Geometry: final body of the model. Coordinates: model frame, mm. A direction names the side the tool comes from. Give positions to 0.01 mm unless a question says otherwise; leave off trailing zeros. Write each loop counter-clockwise with the first axis right and the second up, starting at its lowest first coordinate (ties: lowest second). Pieces come first, ordered by that corner, then holes. Notation, with made-up numbers: (-40, -39) - (-17, -39) arc R28 cw to (-17, -5) - close; hole circle Ø3 at (80, 13.5). An arc over 180 degrees is marked (long way). Use CSV: the item, a comma, the result in double quotes. Start each with the question number.
(1) Line query: probe 1 along Y at (x, z) = (1, 2.3); probe 2 along Y at (x, z) = (3, 0.7); probe 3 along X at (y, z) = (-10.5, 3.85). Output: solid intervals per line, ascending. Write a range as [from, to].
(2) First-contact query: pin 1 Ø12 at (x, y) = (1.5, 9) entering from +Z. Flat tip, straight axial feed; report the tip coordinate or a pass-through.
(3) Draft query along Y for faces 3 (the flat face through (0, 0, 0)), 4 (the cylindrical face through (12.715, 12.699, 2.024)), 5 (the cylindrical face through (3.13, 10.81, 1.98)). Return one class per face: released by +Y, released by -Y, zero draft, split by the parting line, or undercut.
(4) Reachability of faces 1 (the flat face through (0, 13, 2)), 2 (the flat face through (0, 11.2, 2)) from +Z, -Z, +X, -X, +Y, -Y: full face, straight path, thin tool, end or side. Return the list, or none.
(5) Section B-B on x = 0. Output: boundary loops of the cut face in (y, z).
from build123d import *

# Parameters (mm, degrees)
F0_W     = 26
F0_H     = 26
F1_DEPTH = 4
F2_R     = 1
F4_W     = 7
F4_H     = 2.6
F5_DEPTH = 25
F6_R     = 1.29999
F7_R     = 0.3


# Not quite as in the source:
# - a fillet or chamfer is up to 0.001 mm smaller than in the source, because OpenCascade refuses the exact size


with BuildPart() as f1:
    # F0 (on Top) → F1 (new body)
    with BuildSketch(Plane.XY):
        Rectangle(F0_W, F0_H)
    extrude(amount=F1_DEPTH)

    # F2
    f2_edges = [f1.edges().sort_by_distance(p)[0] for p in [
        (-13, -13, 2),
        (-13, 13, 2),
        (13, -13, 2),
        (13, 13, 2),
    ]]
    fillet(f2_edges, radius=F2_R)

    # F4 (on face) → F5 (cut)
    with BuildSketch(Plane.XY.offset(4)):
        with Locations((0, 9.9)):
            Rectangle(F4_W, F4_H)
    extrude(amount=-F5_DEPTH, mode=Mode.SUBTRACT)

    # F6 (radius 1.3 in the source; OpenCascade refuses exactly that, so slightly less here)
    f6_edges = [f1.edges().sort_by_distance(p)[0] for p in [
        (-3.5, 11.2, 2),
        (3.5, 11.2, 2),
        (3.5, 8.6, 2),
        (-3.5, 8.6, 2),
    ]]
    fillet(f6_edges, radius=F6_R)

    # F7
    f7_edges = [f1.edges().sort_by_distance(p)[0] for p in [
        (-13, 0, 4),
        (-13, 0, 0),
        (0, 11.2, 4),
        (0, 11.2, 0),
    ]]
    fillet(f7_edges, radius=F7_R)


solid = f1.part
Check values:
1,probe 1,"y = [-13, 8.6], [11.2, 13]"
1,probe 2,"y = [-13, 8.88], [10.92, 13]"
1,probe 3,"x = [-12.96, 12.96]"
2,pin 1,"stops at z = 4"
3,face 3,"zero draft"
3,face 4,"released by +Y"
3,face 5,"undercut"
4,face 1,"+Z, -Z, +X, -X, +Y"
4,face 2,"+Z, -Z"
5,outline,"(-13, 0.3) arc R0.3 ccw to (-12.7, 0) - (8.3, 0) arc R0.3 ccw to (8.6, 0.3) - (8.6, 3.7) arc R0.3 ccw to (8.3, 4) - (-12.7, 4) arc R0.3 ccw to (-13, 3.7) - close; (11.2, 0.3) arc R0.3 ccw to (11.5, 0) - (12.7, 0) arc R0.3 ccw to (13, 0.3) - (13, 3.7) arc R0.3 ccw to (12.7, 4) - (11.5, 4) arc R0.3 ccw to (11.2, 3.7) - close"
